from build123d import *

# Parameters (mm, degrees)
F0_W      = 50.8
F0_H      = 25.4
F1_DEPTH  = 25.4
F2_W      = 25.4
F2_H      = 12.7
F2_R      = 6.35
F3_DEPTH  = 25.401
F6_DEPTH  = 25.4
F9_DEPTH  = 38.1
F12_DEPTH = 12.7
F14_DEPTH = 6.35
F15_R     = 3.175
F16_DEPTH = 25.4096862922
F17_DEPTH = 38.1322003911


with BuildPart() as f1:
    # F0 (on Front) → F1 (new body)
    with BuildSketch(Plane.XZ):
        with Locations((-0.7526604459, -33.2124557674)):
            Rectangle(F0_W, F0_H)
    extrude(amount=F1_DEPTH)

    # F2 (on face) → F3 (cut, through all)
    with BuildSketch(Plane.XY.offset(-20.5124557674)):
        with Locations((-13.4526604459, -6.35)):
            Rectangle(F2_W, F2_H)
        with Locations((11.9473395541, -12.7)):
            Circle(F2_R)
    extrude(amount=-F3_DEPTH, mode=Mode.SUBTRACT)

    # F5 (on offset) → F6 (join)
    with BuildSketch(Plane(origin=(-0.7526604459, 0, 0), x_dir=(0, -1, 0), z_dir=(-1, 0, 0))):
        Polygon((0, -20.5436561584), (-25.4, 4.8563438416), (-25.4, -33.2436561584), (12.6998899505, -33.2436561584), align=None)
    extrude(amount=-F6_DEPTH)

    # F8 (on offset) → F9 (join)
    with BuildSketch(Plane.XY.offset(4.8875442326)):
        Polygon((-0.7548585206, 50.7596358657), (-0.7548585206, 38.0798179328), (11.9451414794, 38.0798179328), (11.9451414794, 25.3414772451), (24.6538277715, 25.3411643207), (24.6473395541, 50.7596358657), align=None)
    extrude(amount=-F9_DEPTH)

    # F11 (on offset) → F12 (join)
    with BuildSketch(Plane.XY.offset(-45.9124557674)):
        Polygon((24.6473395541, 50.7596358657), (-0.7548585206, 50.7596358657), (-26.1525642636, 50.7596358657), (-26.1525642636, 25.3394645815), (-7.1026604459, 25.4), (-7.1026604459, -12.7), (-0.7526574773, -12.7), (-0.7526574773, 0), (24.6473395541, 0), align=None)
    extrude(amount=F12_DEPTH)

    # F13 (on face) → F14 (join)
    with BuildSketch(Plane.XY.offset(-33.2124557674)):
        Polygon((-13.4525642636, 25.3798217309), (-13.4525642636, 50.7596358657), (-26.1525642636, 50.7596358657), (-26.1525642636, 25.3394645815), align=None)
    extrude(amount=F14_DEPTH)

    # F15 (on face) → F16 (cut, through all)
    with BuildSketch(Plane(origin=(-0.7548585206, 0, 0), x_dir=(0, -1, 0), z_dir=(-1, 0, 0))):
        with Locations((-44.4096358657, -11.8173363179)):
            Circle(F15_R)
    extrude(amount=-F16_DEPTH, mode=Mode.SUBTRACT)

    # F17 (cut, through all): a face of the model
    f17_faces = [f1.faces().sort_by_distance(p)[0] for p in [
        (11.9473395541, -10.0049168283, -33.2436561584),
    ]]
    extrude(f17_faces, amount=-F17_DEPTH, mode=Mode.SUBTRACT)


solid = f1.part
Could you check a few things on this model? Use its own coordinates, in mm. A direction names the side the tool comes from. Round coordinates to 2 decimals unless told otherwise and drop trailing zeros. Order: outer loops, then holes, each group sorted by start corner. A loop starts at its lowest first (then second) coordinate and runs counter-clockwise, first axis right, second up.
(1) If we mould it in two halves opening along Z, with no side actions, what happens to faces 1 (the flat face through (-1, -25.4, -33)), 2 (the flat face through (11.77, 12.522, -8.021)), 3 (the cylindrical face through (11.77, 41.381, -10.864)), 4 (the flat face through (5, 13, -45.912))? For each: released by +Z, released by -Z, zero draft, split by the parting line, or undercut.
Response values:
face 1: zero draft
face 2: released by +Z
face 3: undercut
face 4: released by -Z
(2) Which directions (+Z, -Z, +X, -X, +Y, -Y) give clear straight access to the entire face, cutting with the end or side of a thin tool? Please do faces 5 (the flat face through (15, 41, 4.888)), 6 (the flat face through (-14, -12.7, -33)), 7 (the flat face through (-13.453, 38, -30)).
Response values:
face 5: +Z, +X, -X, +Y, -Y
face 6: +Z, -X
face 7: +Z, +Y
(3) I'm going to push flat-ended pins straight in: pin 1 (12 mm diameter, centred on y = 0.5, z = -15, fed in from -X); pin 2 (6.5 mm diameter, centred on y = 15, z = -42, fed in from -X); pin 3 (4 mm diameter, centred on x = 8, z = -18, fed in from -Y); pin 4 (4 mm diameter, centred on y = 44.41, z = -11.82, fed in from -X). Where does each tip first touch, or does it pass through?
Response values:
pin 1: stops at x = -0.75
pin 2: stops at x = -7.1
pin 3: stops at y = 0.54
pin 4: passes through
(4) Imagine slicing it at B-B (y = -14). Write out the boundary of the cut face in (x, z), plus the area to 3 significant figures.
Response values:
outline: (-26.15, -45.91) - (5.73, -45.91) - (5.73, -20.51) - (-26.15, -20.51) - close; (18.16, -45.91) - (24.65, -45.91) - (24.65, -20.51) - (18.16, -20.51) - close
area: 975 mm2
(5) Imagine slicing it at A-A (z = -31.5). Count the separate pieces of the cut face and the enclosed holes in it, plus the area to 3 significant figures.
Response values:
separate pieces: 2
enclosed holes: 1
area: 2,290 mm2
(6) Imagine slicing it at C-C (x = 13). Write out the boundary of the cut face in (y, z) (3 decimals), plus the area to 3 significant figures.
Response values:
outline: (-25.4, -45.912) - (-18.962, -45.912) - (-18.962, -20.512) - (-25.4, -20.512) - close; (-6.438, -45.912) - (50.76, -45.912) - (50.76, 4.888) - (25.341, 4.888) - (25.341, 4.798) - (0, -20.544) - (0, -20.512) - (-6.438, -20.512) - close; hole circle Ø6.35 at (44.41, -11.817)
area: 2,550 mm2
(7) Please list where these lines run through material, in increasing order: line 1 along Y through (x, z) = (-14, -38.5); line 2 along Z through (x, y) = (10, 31); line 3 along X through (y, z) = (-20.5, -25).
Response values:
line 1: y = -25.4 to -12.7, 25.38 to 50.76
line 2: z = -45.91 to -33.21
line 3: x = -26.15 to 24.65
(8) Imagine slicing it at D-D (x = -19.5). Write out the boundary of the cut face in (y, z), plus the area to 3 significant figures.
Response values:
outline: (-25.4, -45.91) - (-12.7, -45.91) - (-12.7, -20.51) - (-25.4, -20.51) - close; (25.36, -45.91) - (50.76, -45.91) - (50.76, -26.86) - (25.36, -26.86) - close
area: 806 mm2
